from build123d import *

# Parameters (mm, degrees)
F0_W     = 25.4
F0_H     = 25.4
F1_DEPTH = 25.4
F2_W     = 25.4
F2_H     = 76.2
F3_DEPTH = 25.4


with BuildPart() as f1:
    # F0 (on Front) → F1 (new body)
    with BuildSketch(Plane.XZ):
        with Locations((-12.7, -12.7)):
            Rectangle(F0_W, F0_H)
    extrude(amount=F1_DEPTH)

    # F2 (on Front) → F3 (join)
    with BuildSketch(Plane.XZ):
        Polygon((25.4, 0), (0, 0), (0, -25.4), (25.4, -25.4), (50.8, -25.4), (50.8, 0), align=None)
        with Locations((12.7, 38.1)):
            Rectangle(F2_W, F2_H)
    extrude(amount=F3_DEPTH)


solid = f1.part
The model under review builds one solid part; all positions refer to its coordinate system, in mm. A direction names the side the tool comes from. Round coordinates to 2 decimals unless told otherwise and drop trailing zeros. Loops run counter-clockwise (first coordinate to the right, second up) from the corner with the lowest first, then second, coordinate; pieces in that order, holes last. Notation, with made-up numbers: (48, 31) - (85, 31) arc R19 ccw to (85, 51) - close; hole circle Ø4 at (45, 69.25). An arc over 180 degrees is marked (long way). Use CSV: the item, a comma, the result in double quotes.
(1) Take a section at B-B, the plane z = 67.5. Give the boundary of the cut face in (x, y), plus the area to 3 significant figures.
Working result:
outline,"(0, -25.4) - (25.4, -25.4) - (25.4, 0) - (0, 0) - close"
area,"645 mm^2"
(2) For line 1 (X direction, y = -20.75, z = 36); line 2 (Z direction, x = -19, y = -13.25), list the stretches that pass through material, from the lowest coordinate up.
Working result:
line 1,"x = 0 to 25.4"
line 2,"z = -25.4 to 0"
(3) Take a section at A-A, the plane y = -21.75. Give the boundary of the cut face in (x, z).
Working result:
outline,"(-25.4, -25.4) - (50.8, -25.4) - (50.8, 0) - (25.4, 0) - (25.4, 76.2) - (0, 76.2) - (0, 0) - (-25.4, 0) - close"
(4) Machinability: for faces 1 (the flat face through (38, -13, 0)), 2 (the flat face through (0, -13, 39)), 3 (the flat face through (12, -25.4, 15)), which of the approach directions +Z, -Z, +X, -X, +Y, -Y give a long, thin tool a straight path to every point of the face, cutting with its end or side? Answer none if there is none.
Working result:
face 1,"+Z, +X, +Y, -Y"
face 2,"+Z, -X, +Y, -Y"
face 3,"+Z, -Z, +X, -X, -Y"
(5) Clearance check with flat-ended pins moving along their axes: P1, Ø6, axis at x = -7.5, y = -12, coming from the +Z side; P2, Ø10, axis at y = -13, z = 42.5, coming from the -X side; P3, Ø7.5, axis at y = -10, z = 39.5, coming from the +X side. State where each tip first meets the part, or that it passes through.
Working result:
P1,"stops at z = 0"
P2,"stops at x = 0"
P3,"stops at x = 25.4"
(6) Take a section at C-C, the plane x = 39.5. Give the boundary of the cut face in (y, z), plus the area to 3 significant figures.
Working result:
outline,"(-25.4, -25.4) - (0, -25.4) - (0, 0) - (-25.4, 0) - close"
area,"645 mm^2"
